Geometry check sheet. Reference: the model listing, model coordinates, mm. A direction names the side the tool comes from. Give positions to 0.01 mm unless a question says otherwise; leave off trailing zeros. Order: outer loops, then holes, each group sorted by start corner. A loop starts at its lowest first (then second) coordinate and runs counter-clockwise, first axis right, second up.
from build123d import *

# Parameters (mm, degrees)
SKETCH_W                        = 80
SKETCH_H                        = 65
PAD_DEPTH                       = 90
POCKET_DEPTH                    = 65
THICKNESS_T                     = -3
SKETCH002_W                     = 56
SKETCH002_H                     = 79
POCKET001_DEPTH                 = 5
SKETCH003_W                     = 14
SKETCH003_H                     = 14
POCKET002_DEPTH                 = 5
POCKET003_DEPTH                 = 5
SKETCH005_R                     = 1
POCKET004_DEPTH                 = 5
SKETCH005_LINEARPATTERN_2_R     = 1
POCKET004_LINEARPATTERN_2_DEPTH = 5
SKETCH005_LINEARPATTERN_3_R     = 1
POCKET004_LINEARPATTERN_3_DEPTH = 5
SKETCH005_LINEARPATTERN_4_R     = 1
POCKET004_LINEARPATTERN_4_DEPTH = 5
SKETCH005_LINEARPATTERN_5_R     = 1
POCKET004_LINEARPATTERN_5_DEPTH = 5
LINEARPATTERN001_COUNT          = 6
LINEARPATTERN001_PITCH          = 2.8
SKETCH006_W                     = 15
SKETCH006_H                     = 10
POCKET005_DEPTH                 = 5
SKETCH007_W                     = 12.5
SKETCH007_H                     = 6
POCKET006_DEPTH                 = 5
PAD001_DEPTH                    = 4
SKETCH009_W                     = 15
SKETCH009_H                     = 10
PAD002_DEPTH                    = 2
SKETCH010_W                     = 8
SKETCH010_H                     = 3
POCKET007_DEPTH                 = 5
CHAMFER_SIZE                    = 1.5
CHAMFER001_SIZE                 = 1.5
CHAMFER002_SIZE                 = 1.5
SKETCH011_W                     = 16.5
SKETCH011_H                     = 11
SKETCH011_W_2                   = 12.5
SKETCH011_H_2                   = 6
PAD003_DEPTH                    = 2
CHAMFER003_SIZE                 = 1.9
CHAMFER004_SIZE                 = 1
FILLET_R                        = 2
FILLET001_R                     = 3
FILLET002_R                     = 1
SKETCH012_W                     = 2
SKETCH012_H                     = 2
SKETCH012_W_2                   = 5
PAD004_DEPTH                    = 5
CHAMFER005_SIZE                 = 1.99
SKETCH013_R                     = 1.25
POCKET008_DEPTH                 = 7
FILLET003_R                     = 0.75


with BuildPart() as part:
    # Sketch → Pad (new body)
    with BuildSketch(Plane.XY):
        with Locations((20.71249, -6.444686)):
            Rectangle(SKETCH_W, SKETCH_H)
    extrude(amount=PAD_DEPTH)

    # Sketch001 (on Face2 of Pad) → Pocket (cut)
    with BuildSketch(Plane.XZ.offset(38.944686)):
        Polygon((-19.28751, 0), (32.68222, 90), (-19.28751, 90), align=None)
        Polygon((60.71249, 90), (23.196161, 25.019797), (60.71249, 25.019797), align=None)
    extrude(amount=-POCKET_DEPTH, mode=Mode.SUBTRACT)

    # Thickness
    thickness_openings = [part.faces().sort_by_distance(p)[0] for p in [
        (41.954326, -6.444686, 57.509898),
        (41.954326, -6.444686, 25.019797),
    ]]
    offset(amount=THICKNESS_T, openings=thickness_openings)

    # Sketch002 → Pocket001 (cut)
    with BuildSketch(Plane(origin=(-14.46449, 0, 8.352396), x_dir=(0, -1, 0), z_dir=(-0.865991, 0, 0.500059))):
        with Locations((6.444686, 44.855103)):
            Rectangle(SKETCH002_W, SKETCH002_H)
    extrude(amount=-POCKET001_DEPTH, mode=Mode.SUBTRACT)

    # Sketch003 (on Face6 of Pocket001) → Pocket002 (cut)
    with BuildSketch(Plane.XY.offset(90)):
        with Locations((50.71249, 16.055314)):
            Rectangle(SKETCH003_W, SKETCH003_H)
    extrude(amount=-POCKET002_DEPTH, mode=Mode.SUBTRACT)

    # Sketch004 (on Face3 of Pocket002) → Pocket003 (cut)
    with BuildSketch(Plane.XZ.offset(38.944686)):
        Polygon((16.483818, 55.393683), (2.483821, 31.14497), (8.545998, 27.644969), (22.545995, 51.893681), align=None)
    extrude(amount=-POCKET003_DEPTH, mode=Mode.SUBTRACT)

    # Sketch005 (on Face5 of Pocket002) → Pocket004 (cut)
    with BuildSketch(Plane(origin=(0, 26.055314, 0), x_dir=(-1, 0, 0), z_dir=(0, 1, 0))):
        with Locations((-55.71249, 20)):
            Circle(SKETCH005_R)
    pocket004 = extrude(amount=-POCKET004_DEPTH, mode=Mode.SUBTRACT)

    # Sketch005 LinearPattern 2 → Pocket004 LinearPattern 2 (cut)
    with BuildSketch(Plane(origin=(-2.75, 26.055314, 0), x_dir=(-1, 0, 0), z_dir=(0, 1, 0))):
        with Locations((-55.71249, 20)):
            Circle(SKETCH005_LINEARPATTERN_2_R)
    pocket004_linearpattern_2 = extrude(amount=-POCKET004_LINEARPATTERN_2_DEPTH, mode=Mode.SUBTRACT)

    # Sketch005 LinearPattern 3 → Pocket004 LinearPattern 3 (cut)
    with BuildSketch(Plane(origin=(-5.5, 26.055314, 0), x_dir=(-1, 0, 0), z_dir=(0, 1, 0))):
        with Locations((-55.71249, 20)):
            Circle(SKETCH005_LINEARPATTERN_3_R)
    pocket004_linearpattern_3 = extrude(amount=-POCKET004_LINEARPATTERN_3_DEPTH, mode=Mode.SUBTRACT)

    # Sketch005 LinearPattern 4 → Pocket004 LinearPattern 4 (cut)
    with BuildSketch(Plane(origin=(-8.25, 26.055314, 0), x_dir=(-1, 0, 0), z_dir=(0, 1, 0))):
        with Locations((-55.71249, 20)):
            Circle(SKETCH005_LINEARPATTERN_4_R)
    pocket004_linearpattern_4 = extrude(amount=-POCKET004_LINEARPATTERN_4_DEPTH, mode=Mode.SUBTRACT)

    # Sketch005 LinearPattern 5 → Pocket004 LinearPattern 5 (cut)
    with BuildSketch(Plane(origin=(-11, 26.055314, 0), x_dir=(-1, 0, 0), z_dir=(0, 1, 0))):
        with Locations((-55.71249, 20)):
            Circle(SKETCH005_LINEARPATTERN_5_R)
    pocket004_linearpattern_5 = extrude(amount=-POCKET004_LINEARPATTERN_5_DEPTH, mode=Mode.SUBTRACT)

    # LinearPattern001: Pocket004, Pocket004 LinearPattern 2, Pocket004 LinearPattern 3, Pocket004 LinearPattern 4, Pocket004 LinearPattern 5 ×6
    with Locations(*[(0, 0, -i * LINEARPATTERN001_PITCH) for i in range(1, LINEARPATTERN001_COUNT)]):
        add(pocket004, mode=Mode.SUBTRACT)
        add(pocket004_linearpattern_2, mode=Mode.SUBTRACT)
        add(pocket004_linearpattern_3, mode=Mode.SUBTRACT)
        add(pocket004_linearpattern_4, mode=Mode.SUBTRACT)
        add(pocket004_linearpattern_5, mode=Mode.SUBTRACT)

    # Sketch006 (on Face4 of MultiTransform) → Pocket005 (cut)
    with BuildSketch(Plane.YZ.offset(60.71249)):
        with Locations((0.555314, 11)):
            Rectangle(SKETCH006_W, SKETCH006_H)
    extrude(amount=-POCKET005_DEPTH, mode=Mode.SUBTRACT)

    # Sketch007 (on Face3 of Pocket005) → Pocket006 (cut)
    with BuildSketch(Plane.XZ.offset(38.944686)):
        with Locations((49.46249, 6)):
            Rectangle(SKETCH007_W, SKETCH007_H)
    extrude(amount=-POCKET006_DEPTH, mode=Mode.SUBTRACT)

    # Sketch008 (on Face60 of Pocket006) → Pad001 (join)
    with BuildSketch(Plane(origin=(57.71249, 0, 0), x_dir=(0, -1, 0), z_dir=(-1, 0, 0))):
        Polygon((-10.055314, 18), (-10.055314, 6), (-8.055314, 6), (-8.055314, 16), (6.944686, 16), (6.944686, 6), (8.944686, 6), (8.944686, 18), align=None)
    extrude(amount=PAD001_DEPTH)

    # Sketch009 (on Face65 of Pad001) → Pad002 (join)
    with BuildSketch(Plane(origin=(53.71249, 0, 0), x_dir=(0, -1, 0), z_dir=(-1, 0, 0))):
        with Locations((-0.555314, 11)):
            Rectangle(SKETCH009_W, SKETCH009_H)
    extrude(amount=-PAD002_DEPTH)

    # Sketch010 (on Face63 of Pad002) → Pocket007 (cut)
    with BuildSketch(Plane.YZ.offset(55.71249)):
        with Locations((0.555314, 11)):
            Rectangle(SKETCH010_W, SKETCH010_H)
    extrude(amount=-POCKET007_DEPTH, mode=Mode.SUBTRACT)

    # Chamfer
    chamfer_edges = [part.edges().sort_by_distance(p)[0] for p in [
        (60.71249, 0.555314, 16),
        (60.71249, -6.944686, 11),
        (60.71249, 8.055314, 11),
        (60.71249, 0.555314, 6),
    ]]
    chamfer(chamfer_edges, length=CHAMFER_SIZE)

    # Chamfer001
    chamfer001_edges = [part.edges().sort_by_distance(p)[0] for p in [
        (57.71249, 0.555314, 18),
        (57.71249, -8.944686, 12),
        (57.71249, 10.055314, 12),
    ]]
    chamfer(chamfer001_edges, length=CHAMFER001_SIZE)

    # Chamfer002
    chamfer002_edges = [part.edges().sort_by_distance(p)[0] for p in [
        (53.71249, 10.055314, 12),
        (53.71249, -8.944686, 12),
        (53.71249, 0.555314, 18),
    ]]
    chamfer(chamfer002_edges, length=CHAMFER002_SIZE)

    # Sketch011 (on Face32 of Chamfer002) → Pad003 (join)
    with BuildSketch(Plane.XZ.offset(38.944686)):
        with Locations((49.46249, 5.5)):
            Rectangle(SKETCH011_W, SKETCH011_H)
        with Locations((49.46249, 6)):
            Rectangle(SKETCH011_W_2, SKETCH011_H_2, mode=Mode.SUBTRACT)
    extrude(amount=PAD003_DEPTH)

    # Chamfer003
    chamfer003_edges = [part.edges().sort_by_distance(p)[0] for p in [
        (57.71249, -38.944686, 5.5),
        (49.46249, -38.944686, 11),
        (41.21249, -38.944686, 5.5),
    ]]
    chamfer(chamfer003_edges, length=CHAMFER003_SIZE)

    # Chamfer004
    chamfer004_edges = [part.edges().sort_by_distance(p)[0] for p in [
        (19.514907, -38.944686, 53.643682),
        (9.48382, -38.944686, 43.269326),
        (15.545997, -38.944686, 39.769325),
        (5.514909, -38.944686, 29.394969),
    ]]
    chamfer(chamfer004_edges, length=CHAMFER004_SIZE)

    # Fillet
    fillet_edges = [part.edges().sort_by_distance(p)[0] for p in [
        (6.697355, 26.055314, 45),
        (32.68222, -6.444686, 90),
        (6.697355, -38.944686, 45),
    ]]
    fillet(fillet_edges, radius=FILLET_R)

    # Fillet001
    fillet001_edges = [part.edges().sort_by_distance(p)[0] for p in [
        (60.71249, 26.055314, 12.509898),
    ]]
    fillet(fillet001_edges, radius=FILLET001_R)

    # Fillet002
    fillet002_edges = [part.edges().sort_by_distance(p)[0] for p in [
        (60.71249, -38.944686, 12.509898),
    ]]
    fillet(fillet002_edges, radius=FILLET002_R)

    # Sketch012 → Pad004 (join)
    with BuildSketch(Plane.XY.offset(25.019797)):
        with Locations((56.71249, -34.944686)):
            Rectangle(SKETCH012_W, SKETCH012_H)
        with Locations((35.21249, 22.055314)):
            Rectangle(SKETCH012_W_2, SKETCH012_H)
    extrude(amount=-PAD004_DEPTH)

    # Chamfer005
    chamfer005_edges = [part.edges().sort_by_distance(p)[0] for p in [
        (35.21249, 23.055314, 20.019797),
        (56.71249, -35.944686, 20.019797),
    ]]
    chamfer(chamfer005_edges, length=CHAMFER005_SIZE)

    # Sketch013 (on Face8 of Chamfer005) → Pocket008 (cut)
    with BuildSketch(Plane.XY.offset(25.019797)):
        with Locations((58.21249, -36.444686)):
            Circle(SKETCH013_R)
        with Locations((35.21249, 23.555314)):
            Circle(SKETCH013_R)
    extrude(amount=-POCKET008_DEPTH, mode=Mode.SUBTRACT)

    # Fillet003
    fillet003_edges = [part.edges().sort_by_distance(p)[0] for p in [
        (37.71249, 21.055314, 22.519797),
        (37.71249, 23.055314, 22.519797),
        (37.71249, 23.055314, 19.024797),
        (32.71249, 21.055314, 22.519797),
        (32.71249, 23.055314, 22.519797),
        (32.71249, 23.055314, 19.024797),
        (55.71249, -33.944686, 22.519797),
        (57.71249, -33.944686, 22.519797),
        (55.71249, -35.944686, 22.519797),
        (55.71249, -35.944686, 19.024797),
    ]]
    fillet(fillet003_edges, radius=FILLET003_R)


solid = part.part
Item 1: Scan lines: L1, parallel to Z at x = 50, y = -30.5; L2, parallel to Y at x = 11, z = 25.5; L3, parallel to X at y = 24, z = 14. Record each from-to range of solid material in increasing order.
Reported:
L1: z = 0 to 3, 87 to 90
L2: y = -38.94 to -35.94, 23.06 to 26.06
L3: x = -11.2 to 43.8, 45.63 to 46.55, 48.38 to 49.3, 51.13 to 52.05, 53.88 to 54.8, 56.63 to 60.56
Item 2: Gauge pin test, flat ends, axial feed: pin 1 (1.2 mm diameter, centred on x = 50.21, z = 6, fed in from -Y) (3 decimals); pin 2 (12 mm diameter, centred on x = -2, y = -18, fed in from +Z); pin 3 (2.5 mm diameter, centred on x = 50.21, z = 14.4, fed in from -Y); pin 4 (1.2 mm diameter, centred on x = 47.46, z = 8.8, fed in from +Y). Record the tip position at first contact, or that the pin passes through.
Reported:
pin 1: passes through
pin 2: stops at z = 3
pin 3: stops at y = -38.94
pin 4: stops at y = -35.94
Item 3: Sectioned sample at A-A (y = -24.5). Enter the section's corners in (x, z).
Reported:
outline: (-19.29, 0) - (60.71, 0) - (60.71, 25.02) - (57.71, 25.02) - (57.71, 3) - (-14.09, 3) - (-9.19, 11.49) - (-11.79, 12.99) - close; (27.72, 81.4) - (30.32, 79.9) - (34.41, 87) - (58.98, 87) - (60.71, 90) - (33.84, 90) arc R2 ccw to (32.1, 89) - close
Item 4: Sectioned sample at B-B (y = 18.5). Enter the section's corners in (x, z).
Reported:
outline: (-19.29, 0) - (60.71, 0) - (60.71, 25.02) - (57.71, 25.02) - (57.71, 3) - (-14.09, 3) - (-9.19, 11.49) - (-11.79, 12.99) - close; (27.72, 81.4) - (30.32, 79.9) - (34.41, 87) - (43.71, 87) - (43.71, 90) - (33.84, 90) arc R2 ccw to (32.1, 89) - close; (57.71, 87) - (58.98, 87) - (60.71, 90) - (57.71, 90) - close
Item 5: Sectioned sample at C-C (z = 46.5). Give the number of separate pieces and of enclosed holes in the cut face, and give its area (3 significant figures).
Reported:
separate pieces: 3
enclosed holes: 0
area: 151 mm2
Item 6: Set-up check for faces 4 (the flat face through (19.82, -38.44, 54.04)), 5 (the flat face through (57, 8.055, 11)), 6 (the flat face through (55, 1, 6)), 7 (the flat face through (43.712, 16, 89)): record each of +Z, -Z, +X, -X, +Y, -Y from which the full face is reachable in a straight line by a thin tool's end or side.
Reported:
face 4: -Y
face 5: +X
face 6: none
face 7: +Z
Item 7: Draft check along Z on faces 1 (the flat face through (-10.506, -6.053, 12.25)), 2 (the flat face through (21, 26.055, 34)), 3 (the flat face through (6.455, -34.99, 38.582)). Enter one of: released by +Z, released by -Z, zero draft, split by the parting line, or undercut.
Reported:
face 1: released by +Z
face 2: zero draft
face 3: undercut
